Could you check a few things on this model? Use its own coordinates, in mm. A direction names the side the tool comes from. Coordinates: 2 decimals unless noted, no trailing zeros. Write each loop counter-clockwise with the first axis right and the second up, starting at its lowest first coordinate (ties: lowest second). Pieces come first, ordered by that corner, then holes.
Autodesk Inventor part; units mm, degrees
ref_plane "YZ Plane" through (0, 0, 0) normal (1, 0, 0) x (0, 1, 0)
ref_plane "XZ Plane" through (0, 0, 0) normal (0, 1, 0) x (-1, 0, 0)
ref_plane "XY Plane" through (0, 0, 0) normal (0, 0, 1) x (1, 0, 0)
sketch "Esquisse2" plane through (0, 0, 0) normal (0, 1, 0) x (-1, 0, 0)
  circle A0 centre (0, 0) radius 7.975
  dimension "d0" = 15.95
extrude "Extrusion1" add sketch "Esquisse2" along normal blind 15
sketch "Esquisse4" plane through (0, 15, 0) normal (0, 1, 0) x (1, 0, 0)
  circle A0 centre (0, 0) radius 7.975
  circle A1 centre (0, 0) radius 7.975
  arc A2 (-3.2, -7.3048) -> (0, -7.975) centre (0, 0) ccw
  line L0 (-0.0068, -0.0109) -> (-5.0602, -8.1445)
  line L1 (0, -6.3735) -> (0, 5.2233) construction
  line L2 (-3.2, -7.3048) -> (0, -7.975) construction
  line L3 (-3.2, -7.3048) -> (-3.0743, -6.7048)
  line L4 (0, -7.975) -> (0.1257, -7.375)
  arc A3 (0.1257, -7.375) -> (-3.0743, -6.7048) centre (-1.4743, -7.0399) ccw
  line L5 (-3.0743, -6.7048) -> (0.1257, -7.375) construction
  arc A4 (-7.1498, -3.5328) -> (-5.1314, -6.1048) centre (0, 0) ccw
  line L6 (-5.1314, -6.1048) -> (-7.1498, -3.5328) construction
  line L7 (-5.1314, -6.1048) -> (-4.6492, -5.7264)
  line L8 (-7.1498, -3.5328) -> (-6.6676, -3.1544)
  arc A5 (-4.6492, -5.7264) -> (-6.6676, -3.1544) centre (-5.6584, -4.4404) ccw
  line L9 (-4.6492, -5.7264) -> (-6.6676, -3.1544) construction
  line L10 (-5.1314, -6.1048) -> (-3.2, -7.3048) construction
  line L11 (0, 0) -> (-9.6935, -3.168)
  arc A6 (-4.7097, 6.4358) -> (-6.8963, 4.0051) centre (0, 0) ccw
  line L12 (-6.8963, 4.0051) -> (-4.7097, 6.4358) construction
  line L13 (-6.8963, 4.0051) -> (-6.4406, 3.5951)
  line L14 (-4.7097, 6.4358) -> (-4.254, 6.0258)
  arc A7 (-6.4406, 3.5951) -> (-4.254, 6.0258) centre (-5.3473, 4.8105) ccw
  line L15 (-6.4406, 3.5951) -> (-4.254, 6.0258) construction
  arc A8 (-7.7463, 1.8961) -> (-7.8562, -1.3715) centre (0, 0) ccw
  line L16 (-7.7463, 1.8961) -> (-7.8562, -1.3715) construction
  line L17 (-7.7463, 1.8961) -> (-7.1336, 1.8755)
  line L18 (-7.8562, -1.3715) -> (-7.2435, -1.3921)
  arc A9 (-7.2435, -1.3921) -> (-7.1336, 1.8755) centre (-7.1886, 0.2417) ccw
  line L19 (-7.1336, 1.8755) -> (-7.2435, -1.3921) construction
  line L20 (-7.7463, 1.8961) -> (-6.8963, 4.0051) construction
  line L21 (-7.8562, -1.3715) -> (-7.1498, -3.5328) construction
  line L22 (0, 0) -> (-3.9831, 7.4909)
  arc A10 (6.6117, -4.4594) -> (7.8454, -1.4316) centre (0, 0) ccw
  line L23 (7.8454, -1.4316) -> (6.6117, -4.4594) construction
  line L24 (7.8454, -1.4316) -> (7.2777, -1.2003)
  line L25 (6.6117, -4.4594) -> (6.044, -4.228)
  arc A11 (7.2777, -1.2003) -> (6.044, -4.228) centre (6.6609, -2.7142) ccw
  line L26 (7.2777, -1.2003) -> (6.044, -4.228) construction
  arc A12 (7.9306, 0.8406) -> (6.9268, 3.9522) centre (0, 0) ccw
  line L27 (7.9306, 0.8406) -> (6.9268, 3.9522) construction
  line L28 (7.9306, 0.8406) -> (7.3472, 0.6524)
  line L29 (6.9268, 3.9522) -> (6.3434, 3.764)
  arc A13 (6.3434, 3.764) -> (7.3472, 0.6524) centre (6.8453, 2.2082) ccw
  line L30 (7.3472, 0.6524) -> (6.3434, 3.764) construction
  line L31 (7.9306, 0.8406) -> (7.8454, -1.4316) construction
  line L32 (0.5357, 7.957) -> (0.6208, 7.3499)
  arc A14 (-2.617, 6.8962) -> (0.6208, 7.3499) centre (-0.9981, 7.1231) ccw
  line L33 (0.6208, 7.3499) -> (-2.617, 6.8962) construction
  line L34 (0.5357, 7.957) -> (-2.7021, 7.5033) construction
  arc A15 (0.5357, 7.957) -> (-2.7021, 7.5033) centre (0, 0) ccw
  line L35 (-2.7021, 7.5033) -> (-2.617, 6.8962)
  line L36 (2.7595, 7.4824) -> (0.5357, 7.957) construction
  line L37 (2.7595, 7.4824) -> (2.434, 6.9629)
  line L38 (2.434, 6.9629) -> (5.2044, 5.2269) construction
  line L39 (2.7595, 7.4824) -> (5.5299, 5.7463) construction
  arc A16 (5.5299, 5.7463) -> (2.7595, 7.4824) centre (0, 0) ccw
  arc A17 (2.434, 6.9629) -> (5.2044, 5.2269) centre (3.8192, 6.0949) ccw
  line L40 (5.5299, 5.7463) -> (5.2044, 5.2269)
  line L41 (5.5299, 5.7463) -> (6.9268, 3.9522) construction
  line L42 (-4.7097, 6.4358) -> (-2.7021, 7.5033) construction
  line L43 (0, 0) -> (2.483, -17.7205) construction
  arc A18 (2.1919, -7.6679) -> (5.0845, -6.144) centre (0, 0) ccw
  line L44 (5.0845, -6.144) -> (2.1919, -7.6679) construction
  line L45 (5.0845, -6.144) -> (4.7988, -5.6016)
  line L46 (2.1919, -7.6679) -> (1.9062, -7.1255)
  arc A19 (4.7988, -5.6016) -> (1.9062, -7.1255) centre (3.3525, -6.3636) ccw
  line L47 (4.7988, -5.6016) -> (1.9062, -7.1255) construction
  line L48 (6.6117, -4.4594) -> (5.0845, -6.144) construction
  line L49 (2.1919, -7.6679) -> (0, -7.975) construction
  point P0 (-7.7463, 1.8961)
  point P1 (-7.8562, -1.3715)
  point P2 (-4.7097, 6.4358)
  point P3 (0.5357, 7.957)
  point P4 (-2.7021, 7.5033)
  point P5 (5.5299, 5.7463)
  point P6 (2.7595, 7.4824)
  point P7 (7.9306, 0.8406)
  point P8 (6.9268, 3.9522)
  point P9 (6.6117, -4.4594)
  point P10 (7.8454, -1.4316)
  point P11 (-3.2, -7.3048)
  point P12 (0, -7.975)
  point P13 (-7.1498, -3.5328)
  point P14 (-5.1314, -6.1048)
  point P15 (5.0845, -6.144)
  dimension "d14" = 3.2
  dimension "d28" = 0.6
  dimension "d30" = 1.2
extrude "Extrusion6" cut sketch "Esquisse4" against normal blind 15 contours L28 A13 L29 A0 | A0 L25 A11 L24 | L40 A17 L37 A0 | A0 L46 A19 L45 | L32 A14 L35 A0 | A0 L3 A3 L4 | L14 A7 L13 A0 | A0 L8 A5 L7 | L17 A9 L18 A0
sketch "Esquisse6" plane through (0, 15, 0) normal (0, 1, 0) x (1, 0, 0)
  circle A0 centre (0, 0) radius 8
  dimension "d19" = 16
extrude "Extrusion3" add sketch "Esquisse6" along normal blind 1.5
sketch "Esquisse7" plane through (0, 0, 0) normal (0, -1, 0) x (1, 0, 0)
  circle A0 centre (0, 0) radius 8
extrude "Extrusion4" add sketch "Esquisse7" along normal blind 1.5
sketch "Esquisse8" plane through (0, 16.5, 0) normal (0, 1, 0) x (1, 0, 0)
  circle A0 centre (0, 0) radius 4.5
  dimension "d24" = 9
extrude "Extrusion5" cut sketch "Esquisse8" against normal through all
properties part number "Pièce_moteur_courroie_test_3"
1. I want a section at B-B on z = 0. Please give me the cut outline in (x, y) (3 decimals), plus the area to 3 significant figures.
Verdict:
outline: (-8, -1.5) - (-4.5, -1.5) - (-4.5, 16.5) - (-8, 16.5) - (-8, 15) - (-5.572, 15) - (-5.572, 0) - (-8, 0) - close; (4.5, -1.5) - (8, -1.5) - (8, 0) - (7.975, 0) - (7.975, 15) - (8, 15) - (8, 16.5) - (4.5, 16.5) - close
area: 89.2 mm2
2. I want a section at A-A on x = -0.5. Please give me the cut outline in (y, z), plus the area to 3 significant figures.
Verdict:
outline: (-1.5, -7.98) - (0, -7.98) - (0, -5.57) - (15, -5.57) - (15, -7.98) - (16.5, -7.98) - (16.5, -4.47) - (-1.5, -4.47) - close; (-1.5, 4.47) - (16.5, 4.47) - (16.5, 7.98) - (15, 7.98) - (15, 5.73) - (0, 5.73) - (0, 7.98) - (-1.5, 7.98) - close
area: 56.3 mm2
3. On a 3-axis mill with a long thin cutter (end or side, diameter ignored), from which of +Z, -Z, +X, -X, +Y, -Y can I reach the whole of each face in a straight line? I mean faces 1 (the face through (-7.4, 7.4, -2.97)), 2 (the face through (7.97, 7.4, 0.28)), 3 (the face through (5.28, 7.6, -1.74)), 4 (the face through (5.919, 7.395, 5.345)). Say none if no direction works.
Verdict:
face 1: -Z, -X
face 2: +X
face 3: none
face 4: +Z, +X
4. If we mould it in two halves opening along X, with no side actions, what happens to faces 5 (the face through (3.4, -1.5, -3.4)), 6 (the face through (1.1, 7.4, 7.9)), 7 (the face through (2.33, 15, 5.3))? For each: pulls with the +X half, pulls with the -X half, needs draft (parallel to the pull), parting line crosses it, or undercut.
Verdict:
face 5: needs draft
face 6: pulls with the +X half
face 7: undercut
5. Please list where these lines run through material, in increasing order: line 1 along Y through (x, z) = (6, 3); line 2 along Z through (x, y) = (2.5, 5.25); line 3 along X through (y, z) = (7.5, 0) (3 decimals).
Verdict:
line 1: y = -1.5 to 0, 15 to 16.5
line 2: z = -7.57 to -7.07, -5.13 to -3.74, 3.74 to 4.97
line 3: x = -5.572 to -4.5, 4.5 to 7.975
6. For pin 1 (4 mm diameter, centred on y = 11.5, z = 5, fed in from -X); pin 2 (1.5 mm diameter, centred on y = 13.5, z = 1, fed in from +X); pin 3 (1.5 mm diameter, centred on x = -3, y = 4.5, fed in from -Z); pin 4 (8 mm diameter, centred on x = 0, z = 0, fed in from -Y), each with a flat end and sliding along its axis, tell me the tip position at first contact or that it passes through.
Verdict:
pin 1: stops at x = -7.39
pin 2: stops at x = 7.97
pin 3: stops at z = -7.5
pin 4: passes through
